The listing builds one solid part. Answer for the finished solid, in the listing's coordinates (mm). A direction names the side the tool comes from. Give positions to 0.01 mm unless a question says otherwise; leave off trailing zeros. Loops run counter-clockwise (first coordinate to the right, second up) from the corner with the lowest first, then second, coordinate; pieces in that order, holes last. Notation, with made-up numbers: (50.5, 14.25) - (96.5, 14.25) arc R14 cw to (96.5, 24.25) - close; hole circle Ø1 at (32.5, 30.25). An arc over 180 degrees is marked (long way). Answer as CSV lines item,"result". Start each with the question number.
1) A cutting plane is placed at A-A (x = 11.5). Determine the outline of the cut face in (y, z) (3 decimals).
2) A cutting plane is placed at C-C (z = 1). Determine the outline of the cut face in (x, y).
3) A cutting plane is placed at D-D (y = -4). Determine the outline of the cut face in (x, z), and give its area (3 significant figures).
4) For a pull along Z with two mould halves and no side action, classify faces 4 (the face through (-23, -5, 0)), 5 (the face through (-20, 16.65, 22)), 6 (the face through (20.83, 6.66, 19.36)) as pulls with the +Z half, pulls with the -Z half, needs draft (parallel to the pull), parting line crosses it, or undercut.
5) Find the intervals of material crossed by line 1 along X through (y, z) = (-6.5, 4.5); line 2 along Z through (x, y) = (4.5, -11); line 3 along Z through (x, y) = (14, -9.5), in increasing order.
6) A cutting plane is placed at B-B (x = 20). Determine the outline of the cut face in (y, z) (3 decimals), and give its area (3 significant figures).
7) Flat-ended cylindrical pins translate along their axes: pin 1 (6.5 mm diameter, centred on x = -24.5, z = -4, fed in from -Y); pin 2 (6 mm diameter, centred on x = 17.5, y = -11.5, fed in from +Z); pin 3 (1 mm diameter, centred on y = 10.5, z = 6, fed in from +X) (3 decimals); pin 4 (6 mm diameter, centred on x = -5, y = 0, fed in from +Z). Find the tip coordinate at first contact, or state that the pin passes through.
8) For faces 1 (the face through (15, 7, 19)), 2 (the face through (1.3, 7, 14)), 3 (the face through (-26, -13, -4)), determine the directions among +Z, -Z, +X, -X, +Y, -Y from which every point of the face is accessible in a straight line to the end or side of a thin tool.
```python
from build123d import *

# Parameters (mm, degrees)
SKETCH1_W               = 58
SKETCH1_H               = 38.77382393
SKETCH1_W_2             = 42
SKETCH1_H_2             = 21.5
BOSS_EXTRUDE2_DEPTH     = 33.65
CUT_EXTRUDE3_DEPTH      = 69.21502767
SKETCH7_W               = 4
SKETCH7_H               = 9
CUT_EXTRUDE4_DEPTH      = 8
BOSS_EXTRUDE3_DEPTH     = 58
CUT_EXTRUDE5_DEPTH      = 69.21502767
SKETCH10_W              = 5.5
SKETCH10_H              = 7
CUT_EXTRUDE6_DEPTH      = 15
FILLET1_R               = 1
CUT_EXTRUDE7_DEPTH      = 15
CUT_EXTRUDE7_DEPTH_BACK = 20
SKETCH11_R              = 15


with BuildPart() as part:
    # Sketch1 → Boss-Extrude2 (new body)
    with BuildSketch(Plane(origin=(0, -25, 0), x_dir=(1, 0, 0), z_dir=(0, 1, 0))):
        with Locations((0, -6.386911965)):
            Rectangle(SKETCH1_W, SKETCH1_H)
        with Locations((0, -0.25)):
            Rectangle(SKETCH1_W_2, SKETCH1_H_2, mode=Mode.SUBTRACT)
    extrude(amount=BOSS_EXTRUDE2_DEPTH)

    # Sketch6 → Cut-Extrude3 (cut, through all)
    with BuildSketch(Plane(origin=(29, 0, 0), x_dir=(0, 0, -1), z_dir=(1, 0, 0))):
        Polygon((-11, -25), (-4, -13), (9, -13), (13, -10), (13, -25), align=None)
    extrude(amount=-CUT_EXTRUDE3_DEPTH, mode=Mode.SUBTRACT)

    # Sketch7 → Cut-Extrude4 (cut)
    with BuildSketch(Plane.XZ.offset(13)):
        with Locations((-23, -0.5)):
            Rectangle(SKETCH7_W, SKETCH7_H)
    extrude(amount=-CUT_EXTRUDE4_DEPTH, mode=Mode.SUBTRACT)

    # Sketch9 → Boss-Extrude3 (add)
    with BuildSketch(Plane.ZY.offset(29)):
        Polygon((15.77382393, 8.65), (18.77382393, 16.65), (25.77382393, 16.65), (25.77382393, 8.65), align=None)
    extrude(amount=-BOSS_EXTRUDE3_DEPTH)

    # Sketch8 → Cut-Extrude5 (cut, through all)
    with BuildSketch(Plane.ZY.offset(29)):
        Polygon((25.77382393, 10.361106999), (12.77382393, 2.855553499), (12.77382393, -12.155553499), (25.77382393, -19.661106999), (38.77382393, -12.155553499), (38.77382393, 2.855553499), align=None)
    extrude(amount=-CUT_EXTRUDE5_DEPTH, mode=Mode.SUBTRACT)

    # Sketch10 → Cut-Extrude6 (cut)
    with BuildSketch(Plane(origin=(0, 16.65, 0), x_dir=(1, 0, 0), z_dir=(0, 1, 0))):
        with BuildLine():
            Line((-4.2, -12.77382393), (-4.2, -15.123119728))
            ThreePointArc((-4.2, -15.123119728), (-1.45, -14.77382393), (1.3, -15.123119728))
            Line((1.3, -15.123119728), (1.3, -12.77382393))
            Line((1.3, -12.77382393), (-4.2, -12.77382393))
        make_face()
        with BuildLine():
            Line((1.3, -18.77382393), (1.3, -25.77382393))
            Line((1.3, -25.77382393), (9.55, -25.77382393))
            ThreePointArc((9.55, -25.77382393), (8.90224843, -22.054825081), (7.035281374, -18.77382393))
            Line((7.035281374, -18.77382393), (1.3, -18.77382393))
        make_face()
        with BuildLine():
            Line((1.3, -15.123119728), (1.3, -18.77382393))
            Line((1.3, -18.77382393), (7.035281374, -18.77382393))
            ThreePointArc((7.035281374, -18.77382393), (4.456758602, -16.4942656), (1.3, -15.123119728))
        make_face()
        with BuildLine():
            Line((-4.2, -15.123119728), (-4.2, -18.77382393))
            Line((-4.2, -18.77382393), (1.3, -18.77382393))
            Line((1.3, -18.77382393), (1.3, -15.123119728))
            ThreePointArc((1.3, -15.123119728), (-1.45, -14.77382393), (-4.2, -15.123119728))
        make_face()
        with BuildLine():
            Line((-12.45, -25.77382393), (-4.2, -25.77382393))
            Line((-4.2, -25.77382393), (-4.2, -18.77382393))
            Line((-4.2, -18.77382393), (-9.935281374, -18.77382393))
            ThreePointArc((-9.935281374, -18.77382393), (-11.80224843, -22.054825081), (-12.45, -25.77382393))
        make_face()
        with Locations((-1.45, -22.27382393)):
            Rectangle(SKETCH10_W, SKETCH10_H)
        with BuildLine():
            Line((-9.935281374, -18.77382393), (-4.2, -18.77382393))
            Line((-4.2, -18.77382393), (-4.2, -15.123119728))
            ThreePointArc((-4.2, -15.123119728), (-7.356758602, -16.4942656), (-9.935281374, -18.77382393))
        make_face()
    extrude(amount=-CUT_EXTRUDE6_DEPTH, mode=Mode.SUBTRACT)

    # Fillet1
    fillet1_edges = [part.edges().sort_by_distance(p)[0] for p in [
        (-4.2, 5.75277675, 12.77382393),
        (1.3, 5.75277675, 12.77382393),
    ]]
    fillet(fillet1_edges, radius=FILLET1_R)

    # Sketch11 → Cut-Extrude7 (cut, two sides: drawn at the far end of the back side and taken through both)
    with BuildSketch(Plane(origin=(0, 0, 0), x_dir=(0, 0, -1), z_dir=(1, 0, 0)).offset(-CUT_EXTRUDE7_DEPTH_BACK)):
        with Locations((-25.77382393, -4.65)):
            Circle(SKETCH11_R)
    extrude(amount=CUT_EXTRUDE7_DEPTH + CUT_EXTRUDE7_DEPTH_BACK, mode=Mode.SUBTRACT)


solid = part.part
```
Ans:
1,outline,"(-25, 11) - (-7.245, 11) arc R15 cw to (-12.133, 12.774) - (-12.156, 12.774) - (-12.167, 12.793) arc R15 cw to (-19.65, 25.755) - (-19.661, 25.774) - (-25, 25.774) - close; (-11.875, -10.5) - (-10, -13) - (8.65, -13) - (8.65, -10.5) - close; (-2.055, 11) - (8.65, 11) - (8.65, 15.774) - (16.65, 18.774) - (16.65, 25.774) - (10.361, 25.774) - (10.35, 25.755) arc R15 cw to (2.867, 12.793) - (2.856, 12.774) - (2.833, 12.774) arc R15 cw to start"
2,outline,"(-29, -13) - (-25, -13) - (-25, -5) - (-21, -5) - (-21, 8.65) - (-29, 8.65) - close; (21, -13) - (29, -13) - (29, 8.65) - (21, 8.65) - close"
3,outline,"(-29, -13) - (29, -13) - (29, 12.77) - (15, 12.77) - (15, 11) - (21, 11) - (21, -10.5) - (-21, -10.5) - (-21, 11) - (-20, 11) - (-20, 12.77) - (-29, 12.77) - close"
3,area,"530 mm2"
4,face 4,"undercut"
4,face 5,"needs draft"
4,face 6,"pulls with the +Z half"
5,line 1,"-29 to -21, 21 to 29"
5,line 2,"-11.67 to -10.5, 11 to 12.18"
5,line 3,"-13 to -10.5, 11 to 11.58"
6,outline,"(-25, 11) - (8.65, 11) - (8.65, 15.774) - (16.65, 18.774) - (16.65, 25.774) - (10.361, 25.774) - (2.856, 12.774) - (-12.156, 12.774) - (-19.661, 25.774) - (-25, 25.774) - close; (-11.875, -10.5) - (-10, -13) - (8.65, -13) - (8.65, -10.5) - close"
6,area,"321 mm2"
7,pin 1,"y = -13"
7,pin 2,"z = 16.83"
7,pin 3,"through"
7,pin 4,"z = 12.87"
8,face 1,"+Z"
8,face 2,"+Z, +Y"
8,face 3,"-Z, +X, -X, -Y"
